Work out the finished part from the listing and answer in its coordinate system (mm). Face numbers are marked on the shaded views. A direction names the side the tool comes from. Round coordinates to 2 decimals unless told otherwise and drop trailing zeros. Order: outer loops, then holes, each group sorted by start corner. A loop starts at its lowest first (then second) coordinate and runs counter-clockwise, first axis right, second up. Notation, with made-up numbers: (75, 38.5) - (113, 38.5) arc R11 cw to (113, 52.5) - close; hole circle Ø9 at (2.25, -34.75). An arc over 180 degrees is marked (long way). Use CSV: the item, a comma, the result in double quotes.
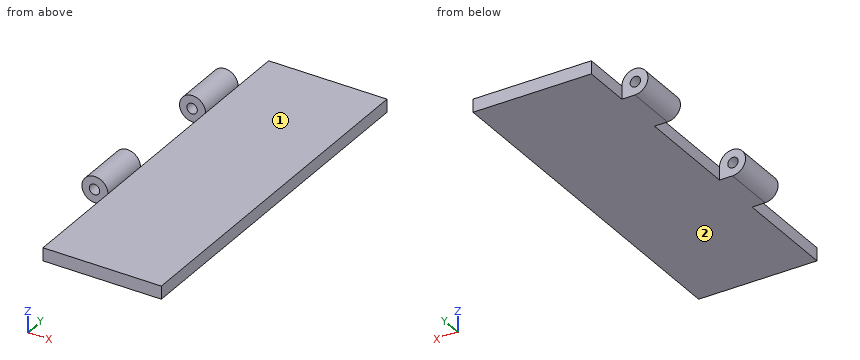
from build123d import *

# Parameters (mm, degrees)
EXTRUDE_1_DEPTH     = 5
EXTRUDE_2_DEPTH     = 20
SKETCH_4_R          = 2
CUT_EXTRUDE_1_DEPTH = 133.533705957


with BuildPart() as part:
    # 草图1 → 凸台-拉伸1 (new body)
    with BuildSketch(Plane.XY):
        Polygon((0, 0), (0, 68.759266336), (-45.494055631, 68.759266336), (-45.494055631, -69.930579597), (0, -69.930579597), align=None)
    extrude(amount=EXTRUDE_1_DEPTH)

    # 草图2 → 凸台-拉伸2 (add)
    with BuildSketch(Plane(origin=(0, 30, 0), x_dir=(1, 0, 0), z_dir=(0, 1, 0))):
        with BuildLine():
            Line((-45.494055631, 0), (-50.502634201, 0))
            ThreePointArc((-50.502634201, 0), (-54.041202389, -8.553225288), (-45.494055631, -5))
            Line((-45.494055631, -5), (-45.494055631, 0))
        make_face()
    extrude_2 = extrude(amount=EXTRUDE_2_DEPTH)

    # 镜向2: 凸台-拉伸2 across plane
    add(extrude_2.mirror(Plane.ZX.offset(10)))

    # 草图4 → 切除-拉伸1 (cut, through all)
    with BuildSketch(Plane(origin=(0, 50, 0), x_dir=(1, 0, 0), z_dir=(0, 1, 0))):
        with Locations(Location((-50.678910059, -4.995787087, 0), (0, 0, 90))):
            Circle(SKETCH_4_R)
    extrude(amount=-CUT_EXTRUDE_1_DEPTH, mode=Mode.SUBTRACT)


solid = part.part
(1) Find section A-A (y = 48.5). Determine the outline of the cut face in (x, z).
Findings below:
outline,"(-50.5, 0) - (0, 0) - (0, 5) - (-45.49, 5) arc R5.01 ccw (long way) to start; hole circle Ø4 at (-50.68, 5)"
(2) Find section B-B (x = -24.5). Determine the outline of the cut face in (y, z), and give its area (3 significant figures).
Findings below:
outline,"(-69.93, 0) - (68.76, 0) - (68.76, 5) - (-69.93, 5) - close"
area,"693 mm²"
(3) For the marked faces 1 and 2, determine the directions among +Z, -Z, +X, -X, +Y, -Y from which every point of the face is accessible in a straight line to the end or side of a thin tool.
Findings below:
face 1,"+Z, +X, +Y, -Y"
face 2,"-Z, +X, -X, +Y, -Y"
(4) Find section C-C (y = 25.5). Determine the outline of the cut face in (x, z), and give its area (3 significant figures).
Findings below:
outline,"(-45.49, 0) - (0, 0) - (0, 5) - (-45.49, 5) - close"
area,"227 mm²"
(5) Each of these flat-tipped pins is pushed along its axis until it touches: pin 1 (1 mm diameter, centred on y = 54, z = 1.5, fed in from -X); pin 2 (3 mm diameter, centred on x = -52, z = 5, fed in from -Y); pin 3 (1 mm diameter, centred on x = -48.5, z = 5, fed in from +Y); pin 4 (5 mm diameter, centred on x = -27.5, y = 41.5, fed in from -Z). Where does it stop, or does it pass through?
Findings below:
pin 1,"stops at x = -45.49"
pin 2,"stops at y = -30"
pin 3,"stops at y = 50"
pin 4,"stops at z = 0"
(6) Find the intervals of material crossed by L1, parallel to Y at x = -52.5, z = 6; L2, parallel to X at y = -17, z = 5.25; L3, parallel to Z at x = -38, y = 19, in increasing order. Write a range as from..to.
Findings below:
L1,"y = -30..-10, 30..50"
L2,"x = -55.51..-52.66, -48.7..-45.5"
L3,"z = 0..5"
